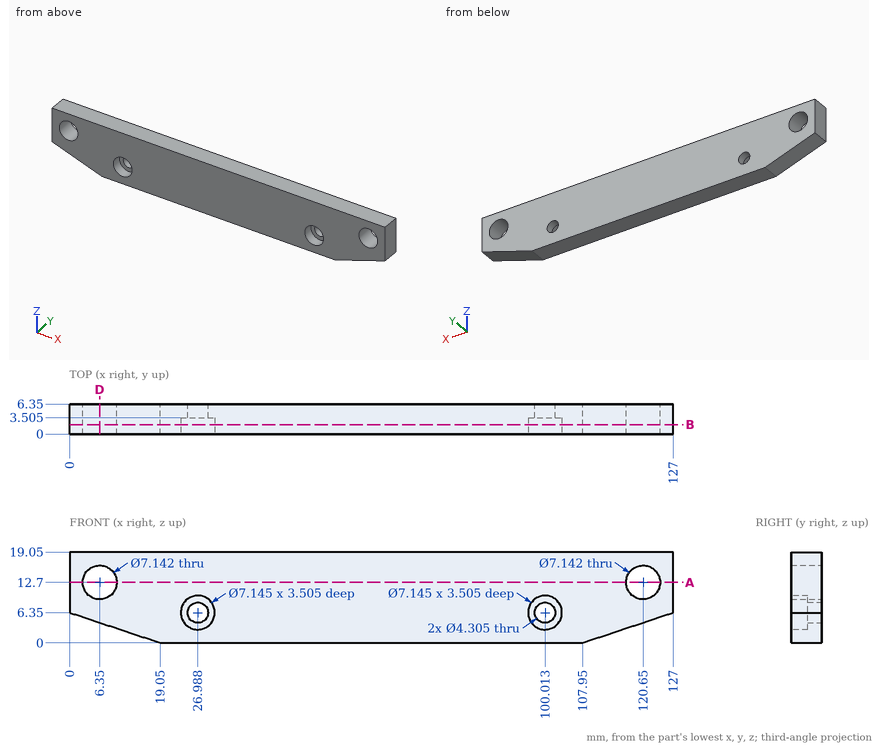
Part print with two shaded views. Sizes in mm from the minimum x, y, z corner. Round coordinates to 2 decimals unless told otherwise and drop trailing zeros. Order: outer loops, then holes, each group sorted by start corner. A loop starts at its lowest first (then second) coordinate and runs counter-clockwise, first axis right, second up. Notation, with made-up numbers: M -18,-23.75 L 16,-23.75 A30 cw 16,-0.75 Z; hole C 2.25,-39.75 d2. An arc over 180 degrees is marked long. Put each result on its own line as item: value. Start each with the question number.
1. Slice it at B-B on y = 2. State how many separate pieces and enclosed holes the cut face has, then the cut area to 3 significant figures.
2. Slice it at A-A on z = 12.7. List the corners of the cut face in (x, y).
3. Drop flat-ended pins along their axis: pin 1 (6.5 mm diameter, centred on x = 120.65, z = 12.7, fed in from +Y); pin 2 (4.5 mm diameter, centred on x = 100.01, z = 6.35, fed in from -Y) (1 decimal); pin 3 (5 mm diameter, centred on x = 26.99, z = 6.35, fed in from +Y). Give the stop position or say it passes through.
4. Slice it at D-D on x = 6.35. List the corners of the cut face in (y, z).
5. Drill centre lines: probe 1 along X at (y, z) = (2, 14.25); probe 2 along X at (y, z) = (2.5, 11.75); probe 3 along X at (y, z) = (1.5, 9.5) (1 decimal). Where is each one in solid material? Low to high. Write a range as [from, to].
Findings:
1. separate pieces: 1
1. enclosed holes: 4
1. area: 2,140 mm2
2. outline: M 0,0 L 2.78,0 L 2.78,6.35 L 0,6.35 Z; M 9.92,0 L 117.08,0 L 117.08,6.35 L 9.92,6.35 Z; M 124.22,0 L 127,0 L 127,6.35 L 124.22,6.35 Z
3. pin 1: through
3. pin 2: y = 3.5
3. pin 3: y = 6.35
4. outline: M 0,4.23 L 6.35,4.23 L 6.35,9.13 L 0,9.13 Z; M 0,16.27 L 6.35,16.27 L 6.35,19.05 L 0,19.05 Z
5. probe 1: [0, 3.13], [9.57, 117.43], [123.87, 127]
5. probe 2: [0, 2.91], [9.79, 117.21], [124.09, 127]
5. probe 3: [0, 4.8], [7.9, 25.3], [28.7, 98.3], [101.7, 119.1], [122.2, 127]
